from build123d import *

# Parameters (mm, degrees)
EXTRUDE_1_DEPTH      = 10
CUT_EXTRUDE_START    = 2.5
CUT_EXTRUDE_1_DEPTH  = 7.5
CUT_EXTRUDE_START_2  = 10
CUT_EXTRUDE_7_DEPTH  = 2.4
CUT_EXTRUDE_START_3  = 2
CUT_EXTRUDE_9_DEPTH  = 8
SKETCH_15_R          = 1.75
CUT_EXTRUDE_10_DEPTH = 10
SKETCH_16_R          = 2.35
CUT_EXTRUDE_11_DEPTH = 6
SKETCH_17_R          = 4
CUT_EXTRUDE_12_DEPTH = 3
FILLET_2_R           = 1
SKETCH_18_R          = 9.75
SKETCH_18_R_2        = 2.55
CUT_EXTRUDE_13_DEPTH = 10


with BuildPart() as part:
    # Эскиз1 → Бобышка-Вытянуть1 (new body)
    with BuildSketch(Plane(origin=(0, 0, 0), x_dir=(1, 0, 0), z_dir=(0, 1, 0))):
        with BuildLine():
            Line((-21, 25), (21, 25))
            ThreePointArc((21, 25), (24.535533906, 23.535533906), (26, 20))
            Line((26, 20), (26, -20))
            ThreePointArc((26, -20), (24.535533906, -23.535533906), (21, -25))
            Line((21, -25), (-21, -25))
            ThreePointArc((-21, -25), (-24.535533906, -23.535533906), (-26, -20))
            Line((-26, -20), (-26, 20))
            ThreePointArc((-26, 20), (-24.535533906, 23.535533906), (-21, 25))
        make_face()
    extrude(amount=EXTRUDE_1_DEPTH)

    # Эскиз2 → Вырез-Вытянуть1 (cut)
    with BuildSketch(Plane(origin=(0, 0, 0), x_dir=(1, 0, 0), z_dir=(0, 1, 0)).offset(CUT_EXTRUDE_START)):
        with BuildLine():
            Line((-13.25, 18.6), (-13.25, 17.75))
            ThreePointArc((-13.25, 17.75), (-14.860912703, 13.860912703), (-18.75, 12.25))
            Line((-18.75, 12.25), (-19.6, 12.25))
            ThreePointArc((-19.6, 12.25), (-21.014213562, 11.664213562), (-21.6, 10.25))
            Line((-21.6, 10.25), (-21.6, -10.25))
            ThreePointArc((-21.6, -10.25), (-21.014213562, -11.664213562), (-19.6, -12.25))
            Line((-19.6, -12.25), (-18.75, -12.25))
            ThreePointArc((-18.75, -12.25), (-14.860912703, -13.860912703), (-13.25, -17.75))
            Line((-13.25, -17.75), (-13.25, -18.6))
            ThreePointArc((-13.25, -18.6), (-12.664213562, -20.014213562), (-11.25, -20.6))
            Line((-11.25, -20.6), (11.25, -20.6))
            ThreePointArc((11.25, -20.6), (12.664213562, -20.014213562), (13.25, -18.6))
            Line((13.25, -18.6), (13.25, -17.75))
            ThreePointArc((13.25, -17.75), (14.860912703, -13.860912703), (18.75, -12.25))
            Line((18.75, -12.25), (19.6, -12.25))
            ThreePointArc((19.6, -12.25), (21.014213562, -11.664213562), (21.6, -10.25))
            Line((21.6, -10.25), (21.6, 10.25))
            ThreePointArc((21.6, 10.25), (21.014213562, 11.664213562), (19.6, 12.25))
            Line((19.6, 12.25), (18.75, 12.25))
            ThreePointArc((18.75, 12.25), (14.860912703, 13.860912703), (13.25, 17.75))
            Line((13.25, 17.75), (13.25, 18.6))
            ThreePointArc((13.25, 18.6), (12.664213562, 20.014213562), (11.25, 20.6))
            Line((11.25, 20.6), (-11.25, 20.6))
            ThreePointArc((-11.25, 20.6), (-12.664213562, 20.014213562), (-13.25, 18.6))
        make_face()
    extrude(amount=CUT_EXTRUDE_1_DEPTH, mode=Mode.SUBTRACT)

    # Эскиз5 → Вырез-Вытянуть7 (cut)
    with BuildSketch(Plane(origin=(0, 0, 0), x_dir=(1, 0, 0), z_dir=(0, 1, 0)).offset(CUT_EXTRUDE_START_2)):
        with BuildLine():
            Line((-16.25, 18.6), (-16.25, 17.75))
            ThreePointArc((-16.25, 17.75), (-16.982233047, 15.982233047), (-18.75, 15.25))
            Line((-18.75, 15.25), (-19.6, 15.25))
            ThreePointArc((-19.6, 15.25), (-23.135533906, 13.785533906), (-24.6, 10.25))
            Line((-24.6, 10.25), (-24.6, -10.25))
            ThreePointArc((-24.6, -10.25), (-23.135533906, -13.785533906), (-19.6, -15.25))
            Line((-19.6, -15.25), (-18.75, -15.25))
            ThreePointArc((-18.75, -15.25), (-16.982233047, -15.982233047), (-16.25, -17.75))
            Line((-16.25, -17.75), (-16.25, -18.6))
            ThreePointArc((-16.25, -18.6), (-14.785533906, -22.135533906), (-11.25, -23.6))
            Line((-11.25, -23.6), (11.25, -23.6))
            ThreePointArc((11.25, -23.6), (14.785533906, -22.135533906), (16.25, -18.6))
            Line((16.25, -18.6), (16.25, -17.75))
            ThreePointArc((16.25, -17.75), (16.982233047, -15.982233047), (18.75, -15.25))
            Line((18.75, -15.25), (19.6, -15.25))
            ThreePointArc((19.6, -15.25), (23.135533906, -13.785533906), (24.6, -10.25))
            Line((24.6, -10.25), (24.6, 10.25))
            ThreePointArc((24.6, 10.25), (23.135533906, 13.785533906), (19.6, 15.25))
            Line((19.6, 15.25), (18.75, 15.25))
            ThreePointArc((18.75, 15.25), (16.982233047, 15.982233047), (16.25, 17.75))
            Line((16.25, 17.75), (16.25, 18.6))
            ThreePointArc((16.25, 18.6), (14.785533906, 22.135533906), (11.25, 23.6))
            Line((11.25, 23.6), (-11.25, 23.6))
            ThreePointArc((-11.25, 23.6), (-14.785533906, 22.135533906), (-16.25, 18.6))
        make_face()
        with BuildLine():
            Line((-14.25, 18.6), (-14.25, 17.75))
            ThreePointArc((-14.25, 17.75), (-15.568019485, 14.568019485), (-18.75, 13.25))
            Line((-18.75, 13.25), (-19.6, 13.25))
            ThreePointArc((-19.6, 13.25), (-21.721320344, 12.371320344), (-22.6, 10.25))
            Line((-22.6, 10.25), (-22.6, -10.25))
            ThreePointArc((-22.6, -10.25), (-21.721320344, -12.371320344), (-19.6, -13.25))
            Line((-19.6, -13.25), (-18.75, -13.25))
            ThreePointArc((-18.75, -13.25), (-15.568019485, -14.568019485), (-14.25, -17.75))
            Line((-14.25, -17.75), (-14.25, -18.6))
            ThreePointArc((-14.25, -18.6), (-13.371320344, -20.721320344), (-11.25, -21.6))
            Line((-11.25, -21.6), (11.25, -21.6))
            ThreePointArc((11.25, -21.6), (13.371320344, -20.721320344), (14.25, -18.6))
            Line((14.25, -18.6), (14.25, -17.75))
            ThreePointArc((14.25, -17.75), (15.568019485, -14.568019485), (18.75, -13.25))
            Line((18.75, -13.25), (19.6, -13.25))
            ThreePointArc((19.6, -13.25), (21.721320344, -12.371320344), (22.6, -10.25))
            Line((22.6, -10.25), (22.6, 10.25))
            ThreePointArc((22.6, 10.25), (21.721320344, 12.371320344), (19.6, 13.25))
            Line((19.6, 13.25), (18.75, 13.25))
            ThreePointArc((18.75, 13.25), (15.568019485, 14.568019485), (14.25, 17.75))
            Line((14.25, 17.75), (14.25, 18.6))
            ThreePointArc((14.25, 18.6), (13.371320344, 20.721320344), (11.25, 21.6))
            Line((11.25, 21.6), (-11.25, 21.6))
            ThreePointArc((-11.25, 21.6), (-13.371320344, 20.721320344), (-14.25, 18.6))
        make_face(mode=Mode.SUBTRACT)
    extrude(amount=-CUT_EXTRUDE_7_DEPTH, mode=Mode.SUBTRACT)

    # Эскиз14 → Вырез-Вытянуть9 (cut)
    with BuildSketch(Plane(origin=(0, 0, 0), x_dir=(1, 0, 0), z_dir=(0, 1, 0)).offset(CUT_EXTRUDE_START_3)):
        with BuildLine():
            Line((21, 23.4), (14.85, 23.4))
            ThreePointArc((14.85, 23.4), (16.616563146, 21.283281573), (17.25, 18.6))
            Line((17.25, 18.6), (17.25, 17.75))
            ThreePointArc((17.25, 17.75), (17.689339828, 16.689339828), (18.75, 16.25))
            Line((18.75, 16.25), (19.6, 16.25))
            ThreePointArc((19.6, 16.25), (22.283281573, 15.616563146), (24.4, 13.85))
            Line((24.4, 13.85), (24.4, 20))
            ThreePointArc((24.4, 20), (23.404163056, 22.404163056), (21, 23.4))
        make_face()
        with BuildLine():
            Line((-21, -23.4), (-14.85, -23.4))
            ThreePointArc((-14.85, -23.4), (-16.616563146, -21.283281573), (-17.25, -18.6))
            Line((-17.25, -18.6), (-17.25, -17.75))
            ThreePointArc((-17.25, -17.75), (-17.689339828, -16.689339828), (-18.75, -16.25))
            Line((-18.75, -16.25), (-19.6, -16.25))
            ThreePointArc((-19.6, -16.25), (-22.283281573, -15.616563146), (-24.4, -13.85))
            Line((-24.4, -13.85), (-24.4, -20))
            ThreePointArc((-24.4, -20), (-23.404163056, -22.404163056), (-21, -23.4))
        make_face()
    extrude(amount=CUT_EXTRUDE_9_DEPTH, mode=Mode.SUBTRACT)

    # Эскиз15 → Вырез-Вытянуть10 (cut)
    with BuildSketch(Plane(origin=(0, 0, 0), x_dir=(1, 0, 0), z_dir=(0, 1, 0))):
        with Locations(Location((-20, 19, 0), (0, 0, 90))):
            Circle(SKETCH_15_R)
        with Locations(Location((20, -19, 0), (0, 0, 90))):
            Circle(SKETCH_15_R)
    extrude(amount=CUT_EXTRUDE_10_DEPTH, mode=Mode.SUBTRACT)

    # Эскиз16 → Вырез-Вытянуть11 (cut)
    with BuildSketch(Plane(origin=(0, 0, 0), x_dir=(1, 0, 0), z_dir=(0, 1, 0))):
        with Locations(Location((-20, 19, 0), (0, 0, 270))):
            Circle(SKETCH_16_R)
        with Locations(Location((20, -19, 0), (0, 0, 270))):
            Circle(SKETCH_16_R)
    extrude(amount=CUT_EXTRUDE_11_DEPTH, mode=Mode.SUBTRACT)

    # Эскиз17 → Вырез-Вытянуть12 (cut)
    with BuildSketch(Plane(origin=(0, 0, 0), x_dir=(1, 0, 0), z_dir=(0, 1, 0))):
        with Locations(Location((-20, 19, 0), (0, 0, 270))):
            Circle(SKETCH_17_R)
        with Locations(Location((20, -19, 0), (0, 0, 270))):
            Circle(SKETCH_17_R)
    extrude(amount=CUT_EXTRUDE_12_DEPTH, mode=Mode.SUBTRACT)

    # Скругление2
    fillet_2_edges = [part.edges().sort_by_distance(p)[0] for p in [
        (0, 0, -25),
        (24.535533906, 0, -23.535533906),
        (26, 0, 0),
        (24.535533906, 0, 23.535533906),
        (0, 0, 25),
        (-24.535533906, 0, 23.535533906),
        (-26, 0, 0),
        (-24.535533906, 0, -23.535533906),
    ]]
    fillet(fillet_2_edges, radius=FILLET_2_R)

    # Эскиз18 → Вырез-Вытянуть13 (cut)
    with BuildSketch(Plane(origin=(0, 0, 0), x_dir=(1, 0, 0), z_dir=(0, 1, 0))):
        with Locations(Location((0, -5, 0), (0, 0, 90))):
            Circle(SKETCH_18_R)
        with Locations(Location((0, 15, 0), (0, 0, 90))):
            Circle(SKETCH_18_R_2)
    extrude(amount=CUT_EXTRUDE_13_DEPTH, mode=Mode.SUBTRACT)


solid = part.part
Can you work these out from the model? Positions are in its coordinate system, mm. A direction names the side the tool comes from. Give positions to 0.01 mm unless a question says otherwise; leave off trailing zeros. Loops run counter-clockwise (first coordinate to the right, second up) from the corner with the lowest first, then second, coordinate; pieces in that order, holes last. Notation, with made-up numbers: M 62.25,22.5 L 79.25,22.5 A31 cw 79.25,61.5 Z; hole C 48,66.25 d5. An arc over 180 degrees is marked long. One line per item, written item: value. Start each with the question number.
1) Thinking about a two-plate mould opening in Z: for faces 3 (the face through (-24.4, 6, 17)), 4 (the face through (0, 10, 21)), 5 (the face through (14.82, 8.82, -22.1)), which applies, +Z half, -Z half, draft (parallel to the pull), parting line (faces both ways), or undercut?
2) If I drill on line 1 (Z direction, x = 8.5, y = 8.25); line 2 (X direction, y = 9.25, z = -7.5); line 3 (X direction, y = 1.4, z = -19), over which ranges is the centre line in solid material (lowest first)? Write a range as [from, to].
3) If we section it at D-D, the plane x = 6: Write out the boundary of the cut face in (y, z).
4) If we section it at B-B, the plane z = 5: Write out the boundary of the cut face in (x, y), and give its area (3 significant figures).
5) If we section it at C-C, the plane y = 4: Give the number of separate pieces and of enclosed holes in the cut face, and give its area (3 significant figures).
6) If we section it at A-A, the plane x = 0: Write out the boundary of the cut face in (y, z).
7) I'm going to push a flat-ended pin straight in: pin 1 (14 mm diameter, centred on x = 3.5, z = 7.5, fed in from +Y). Where does the tip first touch, or does it pass through?
8) On a 3-axis mill with a long thin cutter (end or side, diameter ignored), from which of +Z, -Z, +X, -X, +Y, -Y can I reach the whole of each face in a straight line? I mean faces 1 (the face through (-17.68, 5.94, 16.7)), 2 (the face through (22, 6, 19)). Say none if no direction works.
Completed:
1. face 3: undercut
1. face 4: draft
1. face 5: undercut
2. line 1: z = [-25, -23.6], [-21.6, -20.6], [20.6, 21.6], [23.6, 25]
2. line 2: x = [-26, -24.6], [-22.6, -21.6], [21.6, 22.6], [24.6, 26]
2. line 3: x = [-26, -24], [-16, 26]
3. outline: M 0,-24 A1 ccw 1,-25 L 10,-25 L 10,-23.6 L 7.6,-23.6 L 7.6,-21.6 L 10,-21.6 L 10,-20.6 L 2.5,-20.6 L 2.5,-2.69 L 0,-2.69 Z; M 0,12.69 L 2.5,12.69 L 2.5,20.6 L 10,20.6 L 10,21.6 L 7.6,21.6 L 7.6,23.6 L 10,23.6 L 10,25 L 1,25 A1 ccw 0,24 Z
4. outline: M -26,1 A1 ccw -25,0 L -9.75,0 L -9.75,2.5 L -21.6,2.5 L -21.6,10 L -22.6,10 L -22.6,7.6 L -24.6,7.6 L -24.6,10 L -26,10 Z; M 9.75,0 L 25,0 A1 ccw 26,1 L 26,10 L 24.6,10 L 24.6,7.6 L 22.6,7.6 L 22.6,10 L 21.6,10 L 21.6,2.5 L 9.75,2.5 Z
4. area: 137 mm^2
5. separate pieces: 1
5. enclosed holes: 5
5. area: 914 mm^2
6. outline: M 0,-24 A1 ccw 1,-25 L 10,-25 L 10,-23.6 L 7.6,-23.6 L 7.6,-21.6 L 10,-21.6 L 10,-20.6 L 2.5,-20.6 L 2.5,-17.55 L 0,-17.55 Z; M 0,-12.45 L 2.5,-12.45 L 2.5,-4.75 L 0,-4.75 Z; M 0,14.75 L 2.5,14.75 L 2.5,20.6 L 10,20.6 L 10,21.6 L 7.6,21.6 L 7.6,23.6 L 10,23.6 L 10,25 L 1,25 A1 ccw 0,24 Z
7. pin 1: stops at y = 2.5
8. face 1: +Y
8. face 2: -Y
